Work out the finished part from the listing and answer in its coordinate system (mm). A direction names the side the tool comes from. Coordinates: 2 decimals unless noted, no trailing zeros. Order: outer loops, then holes, each group sorted by start corner. A loop starts at its lowest first (then second) coordinate and runs counter-clockwise, first axis right, second up. Notation, with made-up numbers: (17.5, -13.75) -> (67.5, -13.75) arc R18 cw to (67.5, -9.75) -> close; hole circle Ø6 at (18, -16.75). An arc over 180 degrees is marked (long way). Answer as CSV lines item,"result". Start each with the question number.
Item 1: For a pull along Y with two mould halves and no side action, classify faces 6 (the face through (0, 0, 0)), 7 (the face through (-3.3, -3.3, 2)), 8 (the face through (4.619, -1.915, 4.437)), 9 (the face through (3.2, -3.1, 5.7)) as pulls with the +Y half, pulls with the -Y half, needs draft (parallel to the pull), parting line crosses it, or undercut.
Item 2: Section B-B (z = 1.75) is taken. Write down the section's boundary in (x, y).
Item 3: Section A-A (x = 0) is taken. Write down the section's boundary in (y, z), then the cut area to 4 significant figures.
Item 4: Section C-C (z = 6.25) is taken. Write down the section's boundary in (x, y) (3 decimals), then the cut area to 3 significant figures.
Item 5: Each of these flat-tipped pins is pushed along its axis until it touches: pin 1 Ø0.6 at (x, y) = (-4.5, 0) entering from +Z; pin 2 Ø3 at (x, z) = (1, 6) entering from -Y (3 decimals); pin 3 Ø0.7 at (x, y) = (3.5, 3) entering from +Z. Where does it stop, or does it pass through?
Item 6: Straight lines are drawn through the part: L1, parallel to X at y = 3, z = 0.75; L2, parallel to Y at x = 3.5, z = 5.75. For each, find the intervals that lie inside material, in ascending order.
Item 7: Which of the six approach directions +Z, -Z, +X, -X, +Y, -Y give full straight-line access (tool end or side, diameter ignored) to faces 1 (the face through (-4.5, 0, 5.7)), 2 (the face through (-3.3, 3.3, 2)), 3 (the face through (0, -4.5, 5.7)), 4 (the face through (0, 4.5, 5.7)), 5 (the face through (4.5, 0, 5.7))?
```python
from build123d import *

# Parameters (mm, degrees)
CYLINDER002_R     = 0.5
CYLINDER002_DEPTH = 10
CYLINDER003_R     = 0.5
CYLINDER003_DEPTH = 10
CYLINDER004_R     = 0.5
CYLINDER004_DEPTH = 10
CYLINDER005_R     = 0.5
CYLINDER005_DEPTH = 10
CYLINDER006_R     = 0.5
CYLINDER006_DEPTH = 10
CYLINDER007_R     = 0.5
CYLINDER007_DEPTH = 10
CYLINDER008_R     = 0.5
CYLINDER008_DEPTH = 10
CYLINDER001_R     = 0.5
CYLINDER001_DEPTH = 10
CYLINDER_R        = 5
CYLINDER_DEPTH    = 10
CHAMFER_SIZE      = 1


with BuildPart() as cylinder002:
    # Cylinder002 → Cylinder002 (new body)
    with BuildSketch(Plane(origin=(-5, 0, 2), x_dir=(1, 0, 0), z_dir=(0, 0, 1))):
        Circle(CYLINDER002_R)
    extrude(amount=CYLINDER002_DEPTH)


with BuildPart() as cylinder003:
    # Cylinder003 → Cylinder003 (new body)
    with BuildSketch(Plane(origin=(0, 5, 2), x_dir=(1, 0, 0), z_dir=(0, 0, 1))):
        Circle(CYLINDER003_R)
    extrude(amount=CYLINDER003_DEPTH)


with BuildPart() as cylinder004:
    # Cylinder004 → Cylinder004 (new body)
    with BuildSketch(Plane(origin=(0, -5, 2), x_dir=(1, 0, 0), z_dir=(0, 0, 1))):
        Circle(CYLINDER004_R)
    extrude(amount=CYLINDER004_DEPTH)


with BuildPart() as cylinder005:
    # Cylinder005 → Cylinder005 (new body)
    with BuildSketch(Plane(origin=(3.5, -3.5, 2), x_dir=(1, 0, 0), z_dir=(0, 0, 1))):
        Circle(CYLINDER005_R)
    extrude(amount=CYLINDER005_DEPTH)


with BuildPart() as cylinder006:
    # Cylinder006 → Cylinder006 (new body)
    with BuildSketch(Plane(origin=(-3.5, 3.5, 2), x_dir=(1, 0, 0), z_dir=(0, 0, 1))):
        Circle(CYLINDER006_R)
    extrude(amount=CYLINDER006_DEPTH)


with BuildPart() as cylinder007:
    # Cylinder007 → Cylinder007 (new body)
    with BuildSketch(Plane(origin=(3.5, 3.5, 2), x_dir=(1, 0, 0), z_dir=(0, 0, 1))):
        Circle(CYLINDER007_R)
    extrude(amount=CYLINDER007_DEPTH)


with BuildPart() as cylinder008:
    # Cylinder008 → Cylinder008 (new body)
    with BuildSketch(Plane(origin=(-3.5, -3.5, 2), x_dir=(1, 0, 0), z_dir=(0, 0, 1))):
        Circle(CYLINDER008_R)
    extrude(amount=CYLINDER008_DEPTH)


with BuildPart() as cylinder001:
    # Cylinder001 → Cylinder001 (new body)
    with BuildSketch(Plane(origin=(5, 0, 2), x_dir=(1, 0, 0), z_dir=(0, 0, 1))):
        Circle(CYLINDER001_R)
    extrude(amount=CYLINDER001_DEPTH)


with BuildPart() as cut007:
    # Cylinder → Cylinder (new body)
    with BuildSketch(Plane.XY):
        Circle(CYLINDER_R)
    extrude(amount=CYLINDER_DEPTH)

    # Chamfer
    chamfer_edges = [cut007.edges().sort_by_distance(p)[0] for p in [
        (-5, 0, 10),
    ]]
    chamfer(chamfer_edges, length=CHAMFER_SIZE)

    # Cut: cut Cylinder001
    add(cylinder001.part, mode=Mode.SUBTRACT)

    # Cut001: cut Cylinder008
    add(cylinder008.part, mode=Mode.SUBTRACT)

    # Cut002: cut Cylinder007
    add(cylinder007.part, mode=Mode.SUBTRACT)

    # Cut003: cut Cylinder006
    add(cylinder006.part, mode=Mode.SUBTRACT)

    # Cut004: cut Cylinder005
    add(cylinder005.part, mode=Mode.SUBTRACT)

    # Cut005: cut Cylinder004
    add(cylinder004.part, mode=Mode.SUBTRACT)

    # Cut006: cut Cylinder003
    add(cylinder003.part, mode=Mode.SUBTRACT)

    # Cut007: cut Cylinder002
    add(cylinder002.part, mode=Mode.SUBTRACT)


solid = cut007.part
```
Checked values:
1,face 6,"needs draft"
1,face 7,"undercut"
1,face 8,"parting line crosses it"
1,face 9,"undercut"
2,outline,"circle Ø10 at (0, 0)"
3,outline,"(-5, 0) -> (5, 0) -> (5, 2) -> (4.5, 2) -> (4.5, 9.5) -> (4, 10) -> (-4, 10) -> (-4.5, 9.5) -> (-4.5, 2) -> (-5, 2) -> close"
3,area,"91.75 mm^2"
4,outline,"(-4.975, -0.499) arc R5 ccw to (-3.871, -3.165) arc R0.5 cw (long way) to (-3.165, -3.871) arc R5 ccw to (-0.499, -4.975) arc R0.5 cw to (0.499, -4.975) arc R5 ccw to (3.165, -3.871) arc R0.5 cw (long way) to (3.871, -3.165) arc R5 ccw to (4.975, -0.499) arc R0.5 cw to (4.975, 0.499) arc R5 ccw to (3.871, 3.165) arc R0.5 cw (long way) to (3.165, 3.871) arc R5 ccw to (0.499, 4.975) arc R0.5 cw to (-0.499, 4.975) arc R5 ccw to (-3.165, 3.871) arc R0.5 cw (long way) to (-3.871, 3.165) arc R5 ccw to (-4.975, 0.499) arc R0.5 cw to start"
4,area,"75.3 mm^2"
5,pin 1,"stops at z = 9.8"
5,pin 2,"stops at y = -4.975"
5,pin 3,"stops at z = 9.74"
6,L1,"x = -4 to 4"
6,L2,"y = -3 to 3"
7,face 1,"+Z, -X"
7,face 2,"+Z"
7,face 3,"+Z, -Y"
7,face 4,"+Z, +Y"
7,face 5,"+Z, +X"
